The model under review builds one solid part; all positions refer to its coordinate system, in mm. Face numbers are marked on the shaded views. A direction names the side the tool comes from. Coordinates: 2 decimals unless noted, no trailing zeros. Order: outer loops, then holes, each group sorted by start corner. A loop starts at its lowest first (then second) coordinate and runs counter-clockwise, first axis right, second up.
from build123d import *

# Parameters (mm, degrees)
F0_W           = 20
F0_H           = 20
F1_DEPTH       = 10
F2_R           = 2.0157754343
F3_DEPTH       = 25
F3_DEPTH_BACK  = 25
F5_D           = 5.08
F5_CBORE_D     = 8
F5_CBORE_DEPTH = 5.08
F7_D           = 2
F7_DEPTH       = 4
F7_TIP         = 0.600860619
F9_D           = 2
F9_DEPTH       = 4
F9_TIP         = 0.600860619


with BuildPart() as f1:
    # F0 (on Top) → F1 (new body)
    with BuildSketch(Plane.XY):
        Rectangle(F0_W, F0_H)
    extrude(amount=F1_DEPTH)

    # F2 (on Front) → F3 (cut, two sides)
    with BuildSketch(Plane.XZ) as f3_sk:
        Circle(F2_R)
    extrude(amount=F3_DEPTH, mode=Mode.SUBTRACT)
    extrude(f3_sk.sketch, amount=-F3_DEPTH_BACK, mode=Mode.SUBTRACT)

    # F5 (through all)
    with Locations(Plane.XY.offset(10)):
        with Locations((-4.9497474683, 4.9497474683), (-4.9497474683, -4.9497474683), (4.9497474683, -4.9497474683), (4.9497474683, 4.9497474683)):
            CounterBoreHole(F5_D / 2, F5_CBORE_D / 2, F5_CBORE_DEPTH)

    # F7
    with Locations(Plane.XZ.offset(10)):
        with Locations((0, 8.0078877172), (0, 4.0078877172)):
            Hole(F7_D / 2, depth=F7_DEPTH)
            with Locations((0, 0, -(F7_DEPTH + F7_TIP / 2))):  # 118° drill point
                Cone(0, F7_D / 2, F7_TIP, mode=Mode.SUBTRACT)

    # F9
    with Locations(Plane(origin=(0, 10, 0), x_dir=(-1, 0, 0), z_dir=(0, 1, 0))):
        with Locations((0, 4.0078877172), (0, 8.0078877172)):
            Hole(F9_D / 2, depth=F9_DEPTH)
            with Locations((0, 0, -(F9_DEPTH + F9_TIP / 2))):  # 118° drill point
                Cone(0, F9_D / 2, F9_TIP, mode=Mode.SUBTRACT)


solid = f1.part
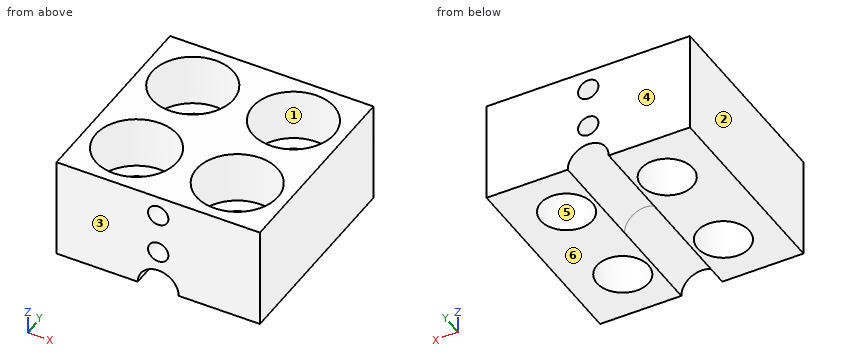
(1) The part is to be moulded in two halves that separate along Y. For the marked faces 3, 4, 5 and 6, say which applies: +Y half, -Y half, draft (parallel to the pull), parting line (faces both ways), or undercut.
(2) Consider section D-D (y = -2). Give the boundary of the cut face in (x, z).
(3) Tool access review of the marked faces 1 and 2: name each direction out of +Z, -Z, +X, -X, +Y, -Y from which nothing blocks a thin tool from reaching the whole face with its end or side.
(4) Consider section B-B (z = 2.5). Give the boundary of the cut face in (x, y).
(5) Insertion check: pin 1 Ø1.2 at (x, z) = (0, 4.01) entering from -Y; pin 2 Ø1.8 at (x, z) = (0, 8.01) entering from +Y; pin 3 Ø6 at (x, y) = (5.5, 5.5) entering from +Z. Each pin has a flat end and moves straight along its axis. Give the tip position at first contact, or say it passes through.
(6) Wall thickness on line 1 (Z direction, x = 0, y = -6.8); line 2 (X direction, y = -5, z = 8.25); line 3 (Y direction, x = -2.75, z = 7.5): over which ranges is each line inside the solid? List them lowest first.
(7) Consider section A-A (x = -5.75). Give the boundary of the cut face in (y, z).
(8) Consider section C-C (y = 3.25). Give the boundary of the cut face in (x, z), then the cut area to 3 significant figures.
Findings:
1. face 3: -Y half
1. face 4: +Y half
1. face 5: undercut
1. face 6: draft
2. outline: (-10, 0) - (-2.02, 0) arc R2.02 cw to (2.02, 0) - (10, 0) - (10, 10) - (7.65, 10) - (7.65, 4.92) - (2.25, 4.92) - (2.25, 10) - (-2.25, 10) - (-2.25, 4.92) - (-7.65, 4.92) - (-7.65, 10) - (-10, 10) - close
3. face 1: +Z
3. face 2: +Z, -Z, -X, +Y, -Y
4. outline: (-10, -10) - (10, -10) - (10, 10) - (-10, 10) - close; hole circle Ø5.08 at (-4.95, -4.95); hole circle Ø5.08 at (-4.95, 4.95); hole circle Ø5.08 at (4.95, -4.95); hole circle Ø5.08 at (4.95, 4.95)
5. pin 1: stops at y = -5.76
5. pin 2: stops at y = 5.94
5. pin 3: stops at z = 4.92
6. line 1: z = 2.02 to 3.01, 5.01 to 7.01, 9.01 to 10
6. line 2: x = -10 to -8.95, -0.95 to 0.95, 8.95 to 10
6. line 3: y = -10 to -8.29, -1.61 to 1.61, 8.29 to 10
7. outline: (-10, 0) - (-7.36, 0) - (-7.36, 4.92) - (-8.87, 4.92) - (-8.87, 10) - (-10, 10) - close; (-2.54, 0) - (2.54, 0) - (2.54, 4.92) - (1.03, 4.92) - (1.03, 10) - (-1.03, 10) - (-1.03, 4.92) - (-2.54, 4.92) - close; (7.36, 0) - (10, 0) - (10, 10) - (8.87, 10) - (8.87, 4.92) - (7.36, 4.92) - close
8. outline: (-10, 0) - (-6.84, 0) - (-6.84, 4.92) - (-8.57, 4.92) - (-8.57, 10) - (-10, 10) - close; (-3.06, 0) - (-2.02, 0) arc R2.02 cw to (2.02, 0) - (3.06, 0) - (3.06, 4.92) - (1.33, 4.92) - (1.33, 10) - (-1.33, 10) - (-1.33, 4.92) - (-3.06, 4.92) - close; (6.84, 0) - (10, 0) - (10, 10) - (8.57, 10) - (8.57, 4.92) - (6.84, 4.92) - close
8. area: 82.9 mm2
